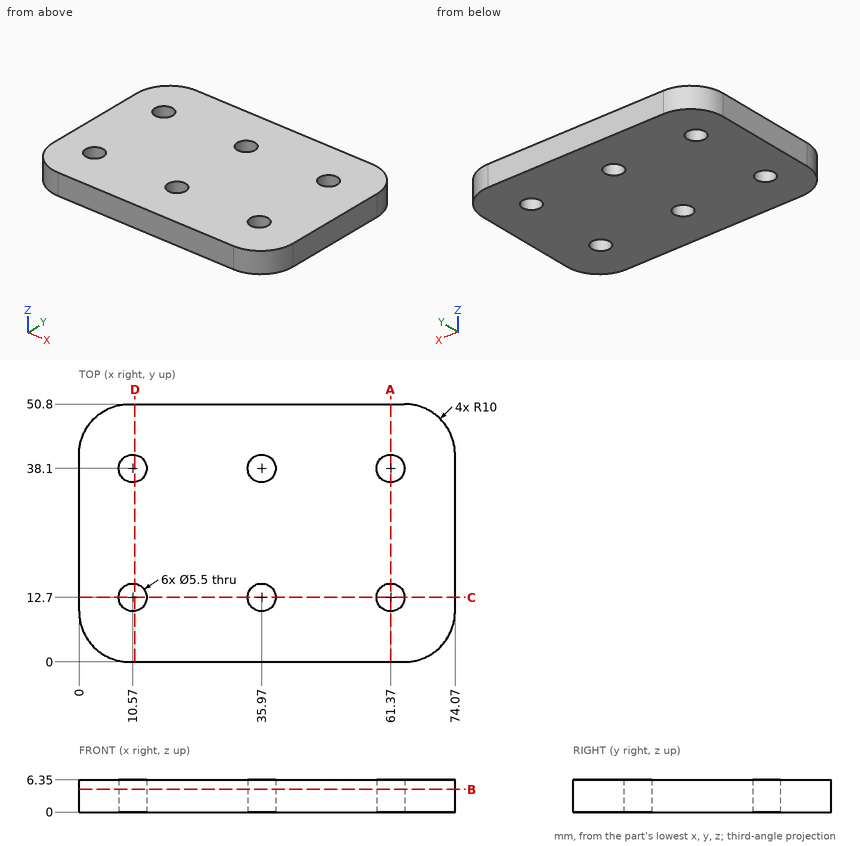
Verification items for this drawing (mm, ordinates from the low corner). Round coordinates to 2 decimals unless told otherwise and drop trailing zeros. Order: outer loops, then holes, each group sorted by start corner. A loop starts at its lowest first (then second) coordinate and runs counter-clockwise, first axis right, second up.
1) Cross-section at A-A, the plane x = 61.37. Record the cut outline in (y, z).
Geometry says:
outline: (0, 0) - (9.95, 0) - (9.95, 6.35) - (0, 6.35) - close; (15.45, 0) - (35.35, 0) - (35.35, 6.35) - (15.45, 6.35) - close; (40.85, 0) - (50.8, 0) - (50.8, 6.35) - (40.85, 6.35) - close
2) Cross-section at D-D, the plane x = 11. Record the cut outline in (y, z), plus the area to 3 significant figures.
Geometry says:
outline: (0, 0) - (9.98, 0) - (9.98, 6.35) - (0, 6.35) - close; (15.42, 0) - (35.38, 0) - (35.38, 6.35) - (15.42, 6.35) - close; (40.82, 0) - (50.8, 0) - (50.8, 6.35) - (40.82, 6.35) - close
area: 254 mm2
3) Material ranges on line 1 (Y direction, x = 61.37, z = 1.5); line 2 (X direction, y = 12.5, z = 3.25); line 3 (X direction, y = 14.5, z = 3.25), recorded low to high.
Geometry says:
line 1: y = 0 to 9.95, 15.45 to 35.35, 40.85 to 50.8
line 2: x = 0 to 7.83, 13.31 to 33.23, 38.71 to 58.63, 64.11 to 74.07
line 3: x = 0 to 8.49, 12.65 to 33.89, 38.05 to 59.29, 63.45 to 74.07
4) Cross-section at B-B, the plane z = 4.5. Record the cut outline in (x, y), plus the area to 3 significant figures.
Geometry says:
outline: (0, 10) arc R10 ccw to (10, 0) - (64.07, 0) arc R10 ccw to (74.07, 10) - (74.07, 40.8) arc R10 ccw to (64.07, 50.8) - (10, 50.8) arc R10 ccw to (0, 40.8) - close; hole circle Ø5.5 at (10.57, 12.7); hole circle Ø5.5 at (10.57, 38.1); hole circle Ø5.5 at (35.97, 12.7); hole circle Ø5.5 at (35.97, 38.1); hole circle Ø5.5 at (61.37, 12.7); hole circle Ø5.5 at (61.37, 38.1)
area: 3,530 mm2
5) Depth check by flat-ended pin: pin 1 (5 mm diameter, centred on x = 35.97, y = 38.1, fed in from -Z). Enter the tip coordinate at first touch or a pass-through.
Geometry says:
pin 1: passes through
6) Cross-section at C-C, the plane y = 12.7. Record the cut outline in (x, z).
Geometry says:
outline: (0, 0) - (7.82, 0) - (7.82, 6.35) - (0, 6.35) - close; (13.32, 0) - (33.22, 0) - (33.22, 6.35) - (13.32, 6.35) - close; (38.72, 0) - (58.62, 0) - (58.62, 6.35) - (38.72, 6.35) - close; (64.12, 0) - (74.07, 0) - (74.07, 6.35) - (64.12, 6.35) - close
